Can you work these out from the drawing? Everything is in mm from the part's minimum corner. Round coordinates to 2 decimals unless told otherwise and drop trailing zeros. Write each loop counter-clockwise with the first axis right and the second up, starting at its lowest first coordinate (ties: lowest second). Pieces come first, ordered by that corner, then holes. Notation, with made-up numbers: (60, 17) -> (69, 17) arc R12 ccw to (69, 31) -> close; hole circle Ø3 at (70.25, 8). An arc over 180 degrees is marked (long way). Put each result on its own line as item: value. Start each with the question number.
1. Suppose I cut it at B-B (x = 3.75). Please give me the cut outline in (y, z).
2. Suppose I cut it at A-A (z = 231.5). Please give me the cut outline in (x, y), then the cut area to 3 significant figures.
3. For pin 1 (5 mm diameter, centred on x = 9.5, z = 155.5, fed in from +Y); pin 2 (3 mm diameter, centred on x = 11.5, z = 222, fed in from +Y); pin 3 (3 mm diameter, centred on y = 8, z = 567, fed in from +X), each with a flat end and sliding along its axis, tell me the tip position at first contact or that it passes through.
4. I need wall thicknesses on probe 1 along Y at (x, z) = (6, 680); probe 2 along X at (y, z) = (5, 794.5); probe 3 along X at (y, z) = (6.25, 782.5). Which ranges of each line are inside material? Lowest first, please. Write a range as from..to.
5. Suppose I cut it at C-C (y = 2). Please give me the cut outline in (x, z).
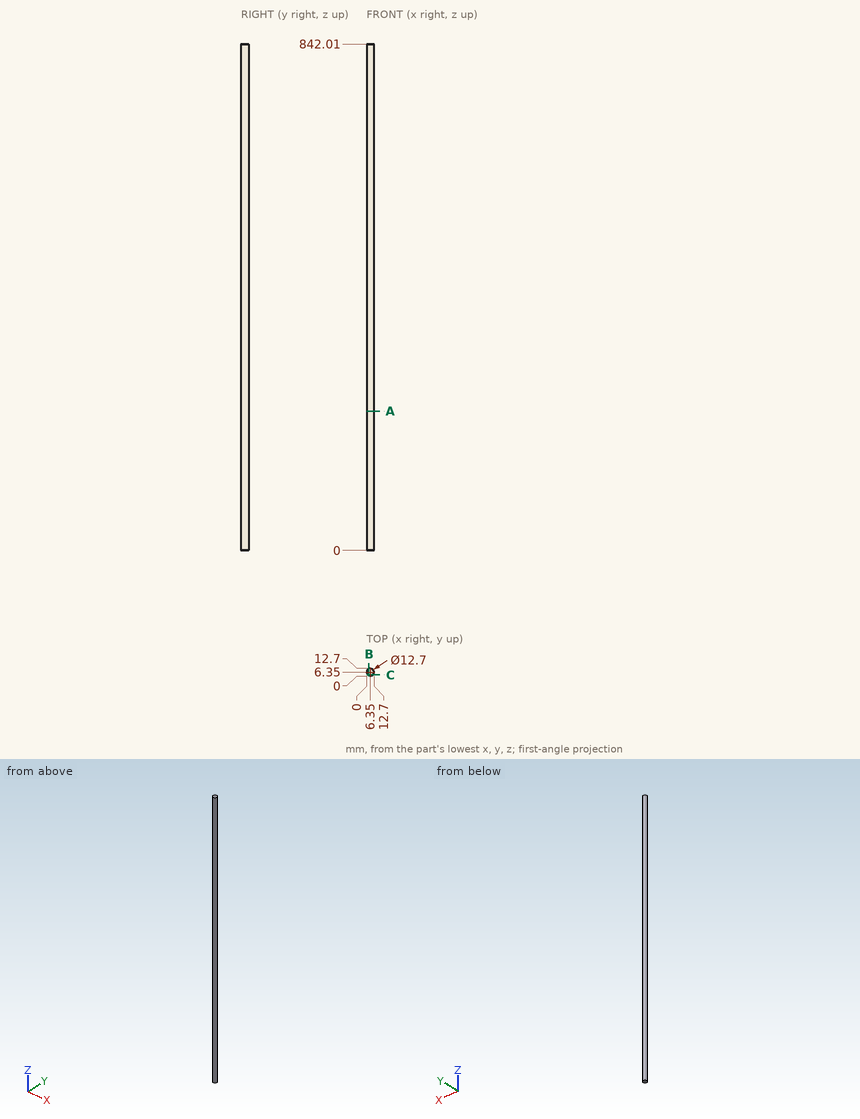
Verdict:
1. outline: (0.56, 0) -> (12.14, 0) -> (12.14, 842.01) -> (0.56, 842.01) -> close
2. outline: circle Ø12.7 at (6.35, 6.35)
2. area: 127 mm^2
3. pin 1: stops at y = 12.67
3. pin 2: stops at y = 11.55
3. pin 3: stops at x = 12.7
4. probe 1: y = 0.01..12.69
4. probe 2: x = 0.15..12.55
4. probe 3: x = 0..12.7
5. outline: (1.72, 0) -> (10.98, 0) -> (10.98, 842.01) -> (1.72, 842.01) -> close
